Can you work these out from the model? Positions are in its coordinate system, mm. Face numbers are marked on the shaded views. A direction names the side the tool comes from. Give positions to 0.01 mm unless a question says otherwise; leave off trailing zeros. Loops run counter-clockwise (first coordinate to the right, second up) from the corner with the lowest first, then second, coordinate; pieces in that order, holes last. Notation, with made-up numbers: (-31.75, -0.5) -> (-4.75, -0.5) arc R14 ccw to (-4.75, 15.5) -> close; hole circle Ø6 at (62.25, 28.5). An arc over 180 degrees is marked (long way). Return JSON: item names as keys, results as strings. Group by question number.
Q1. Suppose I cut it at B-B, the plane y = -14.5. Please give me the cut outline in (x, z) (3 decimals).
Q2. Suppose I cut it at D-D, the plane z = -122.5. Please give me the cut outline in (x, y).
Q3. Will these pins go through, and if not, where does the flat tip stop? pin 1 (9.5 mm diameter, centred on x = -56.5, z = 8, fed in from -Y); pin 2 (1.5 mm diameter, centred on x = 18, z = -10.5, fed in from +Y); pin 3 (5 mm diameter, centred on x = 47.5, z = -60, fed in from +Y); pin 4 (3 mm diameter, centred on x = -40.51, y = -80.84, fed in from -Z).
Q4. Suppose I cut it at A-A, the plane x = -8. Please give me the cut outline in (y, z) (1 decimal).
Q5. Thinking about a two-plate mould opening in X: for the marked faces 1, 2 and 3, which applies, pulls with the +X half, pulls with the -X half, needs draft (parallel to the pull), parting line crosses it, or undercut?
Q6. I need wall thicknesses on line 1 along X through (y, z) = (-17.5, -98); line 2 along Y through (x, z) = (-44.5, -64); line 3 along X through (y, z) = (58.5, -34.5). Which ranges of each line are inside material? Lowest first, please. Write a range as [from, to].
Q7. Which directions (+Z, -Z, +X, -X, +Y, -Y) give clear straight access to the entire face, cutting with the end or side of a thin tool? Please do the marked faces 4, 5 and 6.
Q8. Suppose I cut it at C-C, the plane y = -50. Please give me the cut outline in (x, z) (3 decimals), and give its area (3 significant figures).
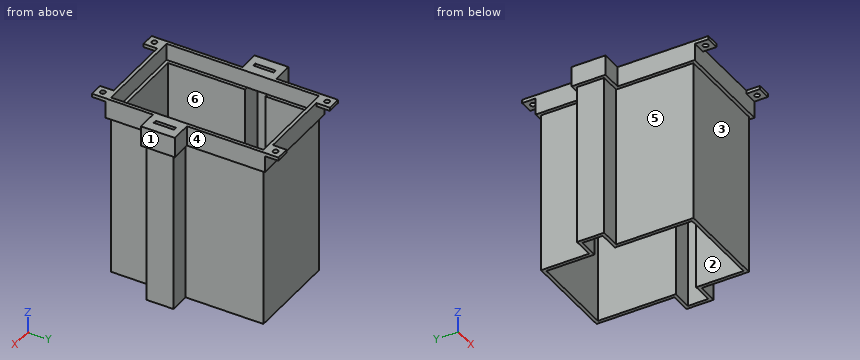
```python
from build123d import *

# Parameters (mm, degrees)
BOSS_EXTRUDE1_DEPTH     = 155.575
SHELL1_T                = -3.175
SKETCH2_W               = 19.05
SKETCH2_H               = 72.263
SKETCH2_H_2             = 44.958
BOSS_EXTRUDE2_DEPTH     = 3.175
SKETCH5_W               = 90.551
SKETCH5_H               = 19.05
BOSS_EXTRUDE8_DEPTH     = 3.175
SKETCH7_W               = 19.05
SKETCH7_H               = 47.498
ALL_6_DEPTH             = 3.175
SKETCH8_W               = 19.05
SKETCH8_H               = 72.898
ALL_5_DEPTH             = 3.175
SKETCH9_W               = 93.726
SKETCH9_H               = 19.05
BOSS_EXTRUDE12_DEPTH    = 3.175
SKETCH10_W              = 15.875
SKETCH10_H              = 19.05
ALL2_DEPTH              = 3.175
SKETCH11_W              = 15.875
SKETCH11_H              = 19.05
ALL_7_DEPTH             = 3.175
SKETCH13_W              = 19.05
SKETCH13_H              = 25.4
ALL_2_DEPTH             = 3.175
SKETCH27_W              = 12.7
SKETCH27_H              = 3.175
BOSS_EXTRUDE29_DEPTH    = 12.7
SKETCH28_R              = 2.38125
CUT_EXTRUDE4_DEPTH      = 227.835119161
MIRROR2_COPY_1_SKETCH_W = 12.7
MIRROR2_COPY_1_SKETCH_H = 3.175
MIRROR2_COPY_1_DEPTH    = 12.7
MIRROR2_COPY_2_SKETCH_R = 2.38125
MIRROR2_COPY_2_DEPTH    = 227.835119161
SKETCH31_W              = 15.875
SKETCH31_H              = 22.225
BOSS_EXTRUDE31_DEPTH    = 3.175
SKETCH87_W              = 19.05
SKETCH87_H              = 31.75
ALL3_DEPTH              = 3.175
SKETCH91_W              = 15.875
SKETCH91_H              = 25.4
ALL_4_DEPTH             = 3.175
CUT_EXTRUDE24_DEPTH     = 201.654704914
SKETCH102_W             = 19.05
SKETCH102_H             = 19.05
BOSS_EXTRUDE58_DEPTH    = 3.175
SKETCH103_W             = 19.05
SKETCH103_H             = 19.05
BOSS_EXTRUDE59_DEPTH    = 3.175
SKETCH105_W             = 15.875
SKETCH105_H             = 25.4
BOSS_EXTRUDE65_DEPTH    = 9.525
SKETCH106_W             = 15.875
SKETCH106_H             = 25.4
BOSS_EXTRUDE66_DEPTH    = 9.525
SKETCH107_W             = 15.875
SKETCH107_H             = 25.4
BOSS_EXTRUDE67_DEPTH    = 6.35
SKETCH108_W             = 15.875
SKETCH108_H             = 25.4
BOSS_EXTRUDE68_DEPTH    = 6.35
SKETCH109_W             = 3.175
SKETCH109_H             = 15.875
BOSS_EXTRUDE69_DEPTH    = 3.175
SKETCH110_W             = 3.175
SKETCH110_H             = 15.875
BOSS_EXTRUDE70_DEPTH    = 3.175
SKETCH111_W             = 3.175
SKETCH111_H             = 15.875
BOSS_EXTRUDE71_DEPTH    = 3.175
SKETCH112_W             = 3.175
SKETCH112_H             = 15.875
BOSS_EXTRUDE72_DEPTH    = 3.175


with BuildPart() as part:
    # Sketch1 → Boss-Extrude1 (new body)
    with BuildSketch(Plane.XY):
        Polygon((-43.688, 71.3105), (43.688, 71.3105), (43.688, -1.5875), (62.738, -1.5875), (62.738, -26.9875), (43.688, -26.9875), (43.688, -71.3105), (-43.688, -71.3105), (-43.688, 0.9525), (-62.738, 0.9525), (-62.738, 26.3525), (-43.688, 26.3525), align=None)
    extrude(amount=-BOSS_EXTRUDE1_DEPTH)

    # Shell1
    shell1_openings = [part.faces().sort_by_distance(p)[0] for p in [
        (0, -0.022879475, 0),
    ]]
    offset(amount=SHELL1_T, openings=shell1_openings, kind=Kind.INTERSECTION)

    # Sketch2 → Boss-Extrude2 (add)
    with BuildSketch(Plane.ZY.offset(43.688)):
        with Locations((6.35, -35.179)):
            Rectangle(SKETCH2_W, SKETCH2_H)
        with Locations((6.35, 48.8315)):
            Rectangle(SKETCH2_W, SKETCH2_H_2)
    extrude(amount=BOSS_EXTRUDE2_DEPTH)

    # Sketch5 → Boss-Extrude8 (add)
    with BuildSketch(Plane.XZ.offset(71.3105)):
        with Locations((-1.5875, 6.35)):
            Rectangle(SKETCH5_W, SKETCH5_H)
    extrude(amount=BOSS_EXTRUDE8_DEPTH)

    # Sketch7 → ALL 6 (add)
    with BuildSketch(Plane(origin=(43.688, 0, 0), x_dir=(0, 0, -1), z_dir=(1, 0, 0))):
        with Locations((-6.35, -50.7365)):
            Rectangle(SKETCH7_W, SKETCH7_H)
    extrude(amount=ALL_6_DEPTH)

    # Sketch8 → ALL 5 (add)
    with BuildSketch(Plane(origin=(43.688, 0, 0), x_dir=(0, 0, -1), z_dir=(1, 0, 0))):
        with Locations((-6.35, 34.8615)):
            Rectangle(SKETCH8_W, SKETCH8_H)
    extrude(amount=ALL_5_DEPTH)

    # Sketch9 → Boss-Extrude12 (add)
    with BuildSketch(Plane(origin=(0, 71.3105, 0), x_dir=(1, 0, 0), z_dir=(0, 1, 0))):
        with Locations((0, -6.35)):
            Rectangle(SKETCH9_W, SKETCH9_H)
    extrude(amount=BOSS_EXTRUDE12_DEPTH)

    # Sketch10 → ALL2 (add)
    with BuildSketch(Plane(origin=(0, -1.5875, 0), x_dir=(1, 0, 0), z_dir=(0, 1, 0))):
        with Locations((54.8005, -6.35)):
            Rectangle(SKETCH10_W, SKETCH10_H)
    extrude(amount=ALL2_DEPTH)

    # Sketch11 → ALL 7 (add)
    with BuildSketch(Plane.XZ.offset(26.9875)):
        with Locations((54.8005, 6.35)):
            Rectangle(SKETCH11_W, SKETCH11_H)
    extrude(amount=ALL_7_DEPTH)

    # Sketch13 → ALL 2 (add)
    with BuildSketch(Plane.ZY.offset(62.738)):
        with Locations((6.35, 13.6525)):
            Rectangle(SKETCH13_W, SKETCH13_H)
    extrude(amount=ALL_2_DEPTH)

    # Sketch27 → Boss-Extrude29 (add)
    with BuildSketch(Plane(origin=(0, 74.4855, -58.6105), x_dir=(1, 0, 0), z_dir=(0, -1, 0))):
        with Locations((40.513, 72.898)):
            Rectangle(SKETCH27_W, SKETCH27_H)
    boss_extrude29 = extrude(amount=-BOSS_EXTRUDE29_DEPTH)

    # Sketch28 → Cut-Extrude4 (cut, through all)
    with BuildSketch(Plane(origin=(0, 58.6105, 15.875), x_dir=(1, 0, 0), z_dir=(0, 0, -1))):
        with Locations(Location((40.513, -22.225, 0), (0, 0, 180))):
            Circle(SKETCH28_R)
    cut_extrude4 = extrude(amount=CUT_EXTRUDE4_DEPTH, mode=Mode.SUBTRACT)

    # Mirror1: Boss-Extrude29, Cut-Extrude4 across plane
    add(boss_extrude29.mirror(Plane(origin=(0, 0, 0), x_dir=(0, 0, 1), z_dir=(1, 0, 0))))
    add(cut_extrude4.mirror(Plane(origin=(0, 0, 0), x_dir=(0, 0, 1), z_dir=(1, 0, 0))), mode=Mode.SUBTRACT)

    # Mirror2: Boss-Extrude29, Cut-Extrude4 across plane
    add(boss_extrude29.mirror(Plane.ZX))
    add(cut_extrude4.mirror(Plane.ZX), mode=Mode.SUBTRACT)

    # Mirror2 copy 1 sketch → Mirror2 copy 1 (add)
    with BuildSketch(Plane(origin=(0, -74.4855, -58.6105), x_dir=(-1, 0, 0), z_dir=(0, 1, 0))):
        with Locations((40.513, 72.898)):
            Rectangle(MIRROR2_COPY_1_SKETCH_W, MIRROR2_COPY_1_SKETCH_H)
    extrude(amount=-MIRROR2_COPY_1_DEPTH)

    # Mirror2 copy 2 sketch → Mirror2 copy 2 (cut, through all)
    with BuildSketch(Plane(origin=(0, -58.6105, 15.875), x_dir=(-1, 0, 0), z_dir=(0, 0, -1))):
        with Locations(Location((40.513, -22.225, 0), (0, 0, 180))):
            Circle(MIRROR2_COPY_2_SKETCH_R)
    extrude(amount=MIRROR2_COPY_2_DEPTH, mode=Mode.SUBTRACT)

    # Sketch31 → Boss-Extrude31 (add)
    with BuildSketch(Plane(origin=(-62.738, 0, 0), x_dir=(0, 0, -1), z_dir=(1, 0, 0))):
        with Locations((-7.9375, 15.24)):
            Rectangle(SKETCH31_W, SKETCH31_H)
    extrude(amount=BOSS_EXTRUDE31_DEPTH)

    # Sketch87 → ALL3 (add)
    with BuildSketch(Plane(origin=(62.738, 0, 0), x_dir=(0, 0, -1), z_dir=(1, 0, 0))):
        with Locations((-6.35, -14.2875)):
            Rectangle(SKETCH87_W, SKETCH87_H)
    extrude(amount=ALL3_DEPTH)

    # Sketch91 → ALL 4 (cut)
    with BuildSketch(Plane(origin=(-59.563, 0, 0), x_dir=(0, 0, -1), z_dir=(1, 0, 0))):
        with Locations((-7.9375, 13.6525)):
            Rectangle(SKETCH91_W, SKETCH91_H)
    extrude(amount=-ALL_4_DEPTH, mode=Mode.SUBTRACT)

    # Sketch101 → Cut-Extrude24 (cut, through all)
    with BuildSketch(Plane.XY.offset(-152.4)):
        Polygon((-40.513, -68.1355), (40.513, -68.1355), (40.513, -23.8125), (59.563, -23.8125), (59.563, -4.7625), (40.513, -4.7625), (40.513, 68.1355), (-40.513, 68.1355), (-40.513, 23.1775), (-59.563, 23.1775), (-59.563, 4.1275), (-40.513, 4.1275), align=None)
    extrude(amount=-CUT_EXTRUDE24_DEPTH, mode=Mode.SUBTRACT)

    # Sketch102 → Boss-Extrude58 (add)
    with BuildSketch(Plane(origin=(0, 26.3525, 0), x_dir=(1, 0, 0), z_dir=(0, 1, 0))):
        with Locations((-56.388, -6.35)):
            Rectangle(SKETCH102_W, SKETCH102_H)
    extrude(amount=BOSS_EXTRUDE58_DEPTH)

    # Sketch103 → Boss-Extrude59 (add)
    with BuildSketch(Plane.XZ.offset(-0.9525)):
        with Locations((-56.388, 6.35)):
            Rectangle(SKETCH103_W, SKETCH103_H)
    extrude(amount=BOSS_EXTRUDE59_DEPTH)

    # Sketch105 → Boss-Extrude65 (add)
    with BuildSketch(Plane(origin=(-43.688, 0, 0), x_dir=(0, 0, -1), z_dir=(1, 0, 0))):
        with Locations((-7.9375, 13.6525)):
            Rectangle(SKETCH105_W, SKETCH105_H)
    extrude(amount=-BOSS_EXTRUDE65_DEPTH)

    # Sketch106 → Boss-Extrude66 (add)
    with BuildSketch(Plane.ZY.offset(-43.688)):
        with Locations((7.9375, -14.2875)):
            Rectangle(SKETCH106_W, SKETCH106_H)
    extrude(amount=-BOSS_EXTRUDE66_DEPTH)

    # Sketch107 → Boss-Extrude67 (add)
    with BuildSketch(Plane.ZY.offset(-62.738)):
        with Locations((7.9375, -14.2875)):
            Rectangle(SKETCH107_W, SKETCH107_H)
    extrude(amount=BOSS_EXTRUDE67_DEPTH)

    # Sketch108 → Boss-Extrude68 (add)
    with BuildSketch(Plane(origin=(-62.738, 0, 0), x_dir=(0, 0, -1), z_dir=(1, 0, 0))):
        with Locations((-7.9375, 13.6525)):
            Rectangle(SKETCH108_W, SKETCH108_H)
    extrude(amount=BOSS_EXTRUDE68_DEPTH)

    # Sketch109 → Boss-Extrude69 (add)
    with BuildSketch(Plane(origin=(0, 0.9525, 0), x_dir=(1, 0, 0), z_dir=(0, 1, 0))):
        with Locations((-54.8005, -7.9375)):
            Rectangle(SKETCH109_W, SKETCH109_H)
    extrude(amount=BOSS_EXTRUDE69_DEPTH)

    # Sketch110 → Boss-Extrude70 (add)
    with BuildSketch(Plane.XZ.offset(-26.3525)):
        with Locations((-54.8005, 7.9375)):
            Rectangle(SKETCH110_W, SKETCH110_H)
    extrude(amount=BOSS_EXTRUDE70_DEPTH)

    # Sketch111 → Boss-Extrude71 (add)
    with BuildSketch(Plane.XZ.offset(1.5875)):
        with Locations((54.8005, 7.9375)):
            Rectangle(SKETCH111_W, SKETCH111_H)
    extrude(amount=BOSS_EXTRUDE71_DEPTH)

    # Sketch112 → Boss-Extrude72 (add)
    with BuildSketch(Plane(origin=(0, -26.9875, 0), x_dir=(1, 0, 0), z_dir=(0, 1, 0))):
        with Locations((54.8005, -7.9375)):
            Rectangle(SKETCH112_W, SKETCH112_H)
    extrude(amount=BOSS_EXTRUDE72_DEPTH)


solid = part.part
```
Ans:
{
 "1": {"outline": "(-46.863, -3.175) -> (-43.688, -3.175) -> (-43.688, -155.575) -> (-40.513, -155.575) -> (-40.513, 0) -> (-43.688, 0) -> (-43.688, 15.875) -> (-46.863, 15.875) -> close; (43.688, 0) -> (53.213, 0) -> (53.213, 15.875) -> (43.688, 15.875) -> close; (56.388, 0) -> (59.563, 0) -> (59.563, -155.575) -> (62.738, -155.575) -> (62.738, -3.175) -> (65.913, -3.175) -> (65.913, 15.875) -> (56.388, 15.875) -> close"},
 "2": {"outline": "(-62.74, 0.95) -> (-43.69, 0.95) -> (-43.69, -71.31) -> (43.69, -71.31) -> (43.69, -26.99) -> (62.74, -26.99) -> (62.74, -1.59) -> (43.69, -1.59) -> (43.69, 71.31) -> (-43.69, 71.31) -> (-43.69, 26.35) -> (-62.74, 26.35) -> close; hole (-59.56, 4.13) -> (-40.51, 4.13) -> (-40.51, -68.14) -> (40.51, -68.14) -> (40.51, -23.81) -> (59.56, -23.81) -> (59.56, -4.76) -> (40.51, -4.76) -> (40.51, 68.14) -> (-40.51, 68.14) -> (-40.51, 23.18) -> (-59.56, 23.18) -> close"},
 "3": {"pin 1": "stops at y = -2.22", "pin 2": "stops at y = 71.31", "pin 3": "stops at y = -1.59", "pin 4": "passes through"},
 "4": {"outline": "(-74.5, -3.2) -> (-71.3, -3.2) -> (-71.3, -155.6) -> (-68.1, -155.6) -> (-68.1, 0) -> (-71.3, 0) -> (-71.3, 15.9) -> (-74.5, 15.9) -> close; (68.1, -155.6) -> (71.3, -155.6) -> (71.3, -3.2) -> (74.5, -3.2) -> (74.5, 15.9) -> (71.3, 15.9) -> (71.3, 0) -> (68.1, 0) -> close"},
 "5": {"face 1": "pulls with the +X half", "face 2": "undercut", "face 3": "needs draft"},
 "6": {"line 1": "x = [-43.69, -40.51], [59.56, 62.74]", "line 2": "y = [0.95, 4.13], [23.18, 26.35]", "line 3": "x = [-43.69, -40.51], [40.51, 43.69]"},
 "7": {"face 4": "+Z, -Z, +X, +Y", "face 5": "-Z, -X, -Y", "face 6": "+Z, -Z"},
 "8": {"outline": "(-46.863, -3.175) -> (-43.688, -3.175) -> (-43.688, -155.575) -> (-40.513, -155.575) -> (-40.513, 0) -> (-43.688, 0) -> (-43.688, 15.875) -> (-46.863, 15.875) -> close; (40.513, -155.575) -> (43.688, -155.575) -> (43.688, -3.175) -> (46.863, -3.175) -> (46.863, 15.875) -> (43.688, 15.875) -> (43.688, 0) -> (40.513, 0) -> close", "area": "1,110 mm^2"}
}
